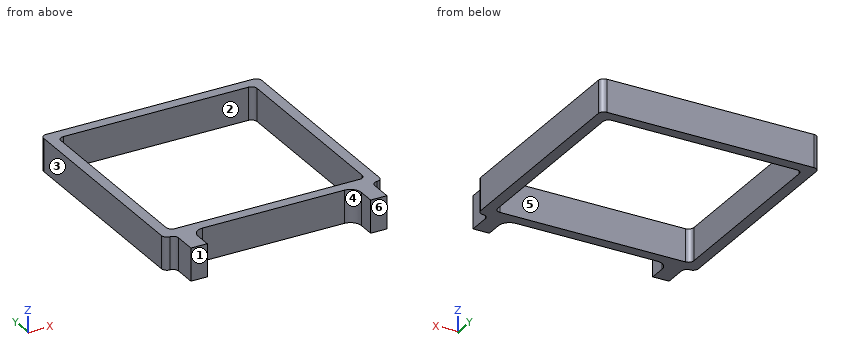
```python
from build123d import *

# Parameters (mm, degrees)
F1_DEPTH = 19.05


with BuildPart() as f1:
    # F0 (on Top) → F1 (new body)
    with BuildSketch(Plane.XY):
        with BuildLine():
            Line((60.325, 63.5), (-60.325, 63.5))
            ThreePointArc((-60.325, 63.5), (-62.570064, 62.570064), (-63.5, 60.325))
            Line((-63.5, 60.325), (-63.5, -60.325))
            ThreePointArc((-63.5, -60.325), (-62.570064, -62.570064), (-60.325, -63.5))
            ThreePointArc((-60.325, -63.5), (-58.079936, -64.429936), (-57.15, -66.675))
            Line((-57.15, -66.675), (-57.15, -79.375))
            Line((-57.15, -79.375), (-47.625, -79.375))
            Line((-47.625, -79.375), (-47.625, -69.85))
            ThreePointArc((-47.625, -69.85), (-45.765128, -65.359872), (-41.275, -63.5))
            Line((-41.275, -63.5), (41.275, -63.5))
            ThreePointArc((41.275, -63.5), (45.765128, -65.359872), (47.625, -69.85))
            Line((47.625, -69.85), (47.625, -79.375))
            Line((47.625, -79.375), (57.15, -79.375))
            Line((57.15, -79.375), (57.15, -66.675))
            ThreePointArc((57.15, -66.675), (58.079936, -64.429936), (60.325, -63.5))
            ThreePointArc((60.325, -63.5), (62.570064, -62.570064), (63.5, -60.325))
            Line((63.5, -60.325), (63.5, 60.325))
            ThreePointArc((63.5, 60.325), (62.570064, 62.570064), (60.325, 63.5))
        make_face()
        with BuildLine():
            ThreePointArc((-57.15, 53.975), (-56.220064, 56.220064), (-53.975, 57.15))
            Line((-53.975, 57.15), (53.975, 57.15))
            ThreePointArc((53.975, 57.15), (56.220064, 56.220064), (57.15, 53.975))
            Line((57.15, 53.975), (57.15, -53.975))
            ThreePointArc((57.15, -53.975), (56.220064, -56.220064), (53.975, -57.15))
            Line((53.975, -57.15), (-53.975, -57.15))
            ThreePointArc((-53.975, -57.15), (-56.220064, -56.220064), (-57.15, -53.975))
            Line((-57.15, -53.975), (-57.15, 53.975))
        make_face(mode=Mode.SUBTRACT)
    extrude(amount=F1_DEPTH)


solid = f1.part
```
Verification items for the finished model (mm, model axes). Face numbers are marked on the shaded views. A direction names the side the tool comes from. Coordinates: 2 decimals unless noted, no trailing zeros. Write each loop counter-clockwise with the first axis right and the second up, starting at its lowest first coordinate (ties: lowest second). Pieces come first, ordered by that corner, then holes. Notation, with made-up numbers: (85.5, 78.25) - (90.5, 78.25) arc R32 cw to (90.5, 110.25) - close; hole circle Ø2 at (-18.5, 88.5). An arc over 180 degrees is marked (long way). Write item = value, one per line.
Q1. Cross-section at C-C (z = 3.75). Enter the section's corners in (x, y) (3 decimals).
Answer:
outline = (-63.5, -60.325) arc R3.175 ccw to (-60.325, -63.5) arc R3.175 cw to (-57.15, -66.675) - (-57.15, -79.375) - (-47.625, -79.375) - (-47.625, -69.85) arc R6.35 cw to (-41.275, -63.5) - (41.275, -63.5) arc R6.35 cw to (47.625, -69.85) - (47.625, -79.375) - (57.15, -79.375) - (57.15, -66.675) arc R3.175 cw to (60.325, -63.5) arc R3.175 ccw to (63.5, -60.325) - (63.5, 60.325) arc R3.175 ccw to (60.325, 63.5) - (-60.325, 63.5) arc R3.175 ccw to (-63.5, 60.325) - close; hole (-57.15, -53.975) arc R3.175 ccw to (-53.975, -57.15) - (53.975, -57.15) arc R3.175 ccw to (57.15, -53.975) - (57.15, 53.975) arc R3.175 ccw to (53.975, 57.15) - (-53.975, 57.15) arc R3.175 ccw to (-57.15, 53.975) - close
Q2. Mould release check, pull along X, two halves, no side actions. Record for the marked faces 1, 2 and 3: released by +X, released by -X, zero draft, split by the parting line, or undercut.
Answer:
face_1 = zero draft
face_2 = undercut
face_3 = released by -X
Q3. Access from +Z, -Z, +X, -X, +Y, -Y to the whole of each face (thin tool, end or side, straight path). Record for the marked faces 4, 5 and 6.
Answer:
face_4 = +Z, -Z, -Y
face_5 = +Z, -Z
face_6 = +Z, -Z, +X, -X, -Y
Q4. Cross-section at B-B (x = 50). Enter the section's corners in (y, z) (3 decimals), plus the area to 3 significant figures.
Answer:
outline = (-79.375, 0) - (-57.15, 0) - (-57.15, 19.05) - (-79.375, 19.05) - close; (57.15, 0) - (63.5, 0) - (63.5, 19.05) - (57.15, 19.05) - close
area = 544 mm²
Q5. Material ranges on L1, parallel to Y at x = -53.5, z = 16.5 (3 decimals); L2, parallel to Y at x = -37, z = 7.5, recorded low to high. Write a range as from..to.
Answer:
L1 = -79.375..-57.15, 57.15..63.5
L2 = -63.5..-57.15, 57.15..63.5
Q6. Go/stop test with flat-tipped pins: pin 1 Ø5 at (y, z) = (-75.5, 12) entering from +X; pin 2 Ø7.5 at (y, z) = (-75, 7) entering from -X; pin 3 Ø1 at (x, z) = (-36.5, 12) entering from -Y. Record where each tip stops, or that it passes through.
Answer:
pin_1 = 57.15
pin_2 = -57.15
pin_3 = -63.5
Q7. Cross-section at A-A (y = 36.5). Enter the section's corners in (x, z).
Answer:
outline = (-63.5, 0) - (-57.15, 0) - (-57.15, 19.05) - (-63.5, 19.05) - close; (57.15, 0) - (63.5, 0) - (63.5, 19.05) - (57.15, 19.05) - close
